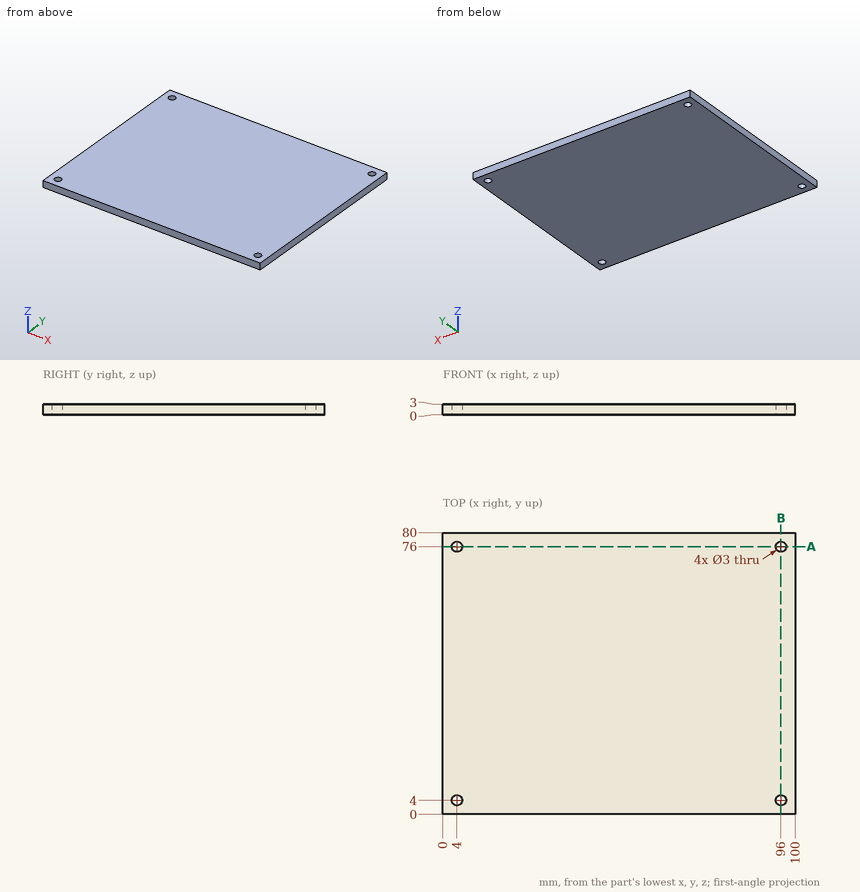
Here's the drawing with two shaded views (mm, measured from the low corner). I have some questions. Coordinates: 2 decimals unless noted, no trailing zeros. Order: outer loops, then holes, each group sorted by start corner. A loop starts at its lowest first (then second) coordinate and runs counter-clockwise, first axis right, second up.
Q1. Suppose I cut it at A-A on y = 76. Please give me the cut outline in (x, z).
Q2. Will this pin go through, and if not, where does the flat tip stop? pin 1 (4 mm diameter, centred on x = 96, y = 4, fed in from +Z).
Q3. Please list where these lines run through material, in increasing order: L1, parallel to Y at x = 4, z = 0.9; L2, parallel to X at y = 4, z = 1.75.
Q4. Suppose I cut it at B-B on x = 96. Please give me the cut outline in (y, z).
Answer:
1. outline: (0, 0) - (2.5, 0) - (2.5, 3) - (0, 3) - close; (5.5, 0) - (94.5, 0) - (94.5, 3) - (5.5, 3) - close; (97.5, 0) - (100, 0) - (100, 3) - (97.5, 3) - close
2. pin 1: stops at z = 3
3. L1: y = 0 to 2.5, 5.5 to 74.5, 77.5 to 80
3. L2: x = 0 to 2.5, 5.5 to 94.5, 97.5 to 100
4. outline: (0, 0) - (2.5, 0) - (2.5, 3) - (0, 3) - close; (5.5, 0) - (74.5, 0) - (74.5, 3) - (5.5, 3) - close; (77.5, 0) - (80, 0) - (80, 3) - (77.5, 3) - close
